from build123d import *

# Parameters (mm, degrees)
SKETCH1_W           = 121.3
SKETCH1_H           = 76.24
BOSS_EXTRUDE1_DEPTH = 7.4
SKETCH2_R           = 2.75
SKETCH2_R_2         = 1.5
BOSS_EXTRUDE2_DEPTH = 5.5
SKETCH3_R           = 2.75
SKETCH3_R_2         = 1.5
BOSS_EXTRUDE3_DEPTH = 5.3
SKETCH4_W           = 108
SKETCH4_H           = 65
CUT_EXTRUDE1_DEPTH  = 0.2
SKETCH5_R           = 8
BOSS_EXTRUDE4_DEPTH = 4
SKETCH6_W           = 5
SKETCH6_H           = 22
BOSS_EXTRUDE5_DEPTH = 3


with BuildPart() as part:
    # Sketch1 → Boss-Extrude1 (new body)
    with BuildSketch(Plane(origin=(0, 0, 0), x_dir=(1, 0, 0), z_dir=(0, 1, 0))):
        Rectangle(SKETCH1_W, SKETCH1_H)
    extrude(amount=BOSS_EXTRUDE1_DEPTH)

    # Sketch2 → Boss-Extrude2 (add)
    # profile 1 of 4: a face of its own
    with BuildSketch(Plane.XZ):
        with Locations(Location((-56.5, 34, 0), (0, 0, 270))):
            Circle(SKETCH2_R)
        with Locations(Location((-56.5, 34, 0), (0, 0, 270))):
            Circle(SKETCH2_R_2, mode=Mode.SUBTRACT)
    # profile 2 of 4: a face of its own
    with BuildSketch(Plane.XZ):
        with Locations(Location((56.5, 34, 0), (0, 0, 270))):
            Circle(SKETCH2_R)
        with Locations(Location((56.5, 34, 0), (0, 0, 270))):
            Circle(SKETCH2_R_2, mode=Mode.SUBTRACT)
    # profile 3 of 4: a face of its own
    with BuildSketch(Plane.XZ):
        with Locations(Location((56.5, -34, 0), (0, 0, 270))):
            Circle(SKETCH2_R)
        with Locations(Location((56.5, -34, 0), (0, 0, 270))):
            Circle(SKETCH2_R_2, mode=Mode.SUBTRACT)
    # profile 4 of 4: a face of its own
    with BuildSketch(Plane.XZ):
        with Locations(Location((-56.5, -34, 0), (0, 0, 270))):
            Circle(SKETCH2_R)
        with Locations(Location((-56.5, -34, 0), (0, 0, 270))):
            Circle(SKETCH2_R_2, mode=Mode.SUBTRACT)
    extrude(amount=BOSS_EXTRUDE2_DEPTH)

    # Sketch3 → Boss-Extrude3 (add)
    # profile 1 of 4: a face of its own
    with BuildSketch(Plane.XZ):
        with Locations(Location((-29.35, 24.62, 0), (0, 0, 270))):
            Circle(SKETCH3_R)
        with Locations(Location((-29.35, 24.62, 0), (0, 0, 270))):
            Circle(SKETCH3_R_2, mode=Mode.SUBTRACT)
    # profile 2 of 4: a face of its own
    with BuildSketch(Plane.XZ):
        with Locations(Location((28.65, 24.62, 0), (0, 0, 270))):
            Circle(SKETCH3_R)
        with Locations(Location((28.65, 24.62, 0), (0, 0, 270))):
            Circle(SKETCH3_R_2, mode=Mode.SUBTRACT)
    # profile 3 of 4: a face of its own
    with BuildSketch(Plane.XZ):
        with Locations(Location((28.65, -24.38, 0), (0, 0, 270))):
            Circle(SKETCH3_R)
        with Locations(Location((28.65, -24.38, 0), (0, 0, 270))):
            Circle(SKETCH3_R_2, mode=Mode.SUBTRACT)
    # profile 4 of 4: a face of its own
    with BuildSketch(Plane.XZ):
        with Locations(Location((-29.35, -24.38, 0), (0, 0, 270))):
            Circle(SKETCH3_R)
        with Locations(Location((-29.35, -24.38, 0), (0, 0, 270))):
            Circle(SKETCH3_R_2, mode=Mode.SUBTRACT)
    extrude(amount=BOSS_EXTRUDE3_DEPTH)

    # Sketch4 → Cut-Extrude1 (cut)
    with BuildSketch(Plane(origin=(0, 7.4, 0), x_dir=(1, 0, 0), z_dir=(0, 1, 0))):
        with Locations((0, 2.62)):
            Rectangle(SKETCH4_W, SKETCH4_H)
    extrude(amount=-CUT_EXTRUDE1_DEPTH, mode=Mode.SUBTRACT)

    # Sketch5 → Boss-Extrude4 (add)
    with BuildSketch(Plane(origin=(0, 0, 0), x_dir=(-1, 0, 0), z_dir=(0, -1, 0))):
        with Locations(Location((43.65, 30.12, 0), (0, 0, 90))):
            Circle(SKETCH5_R)
    extrude(amount=BOSS_EXTRUDE4_DEPTH)

    # Sketch6 → Boss-Extrude5 (add)
    with BuildSketch(Plane.XZ):
        with Locations((-45.15, -3.52)):
            Rectangle(SKETCH6_W, SKETCH6_H)
    extrude(amount=BOSS_EXTRUDE5_DEPTH)


solid = part.part
The model under review builds one solid part; all positions refer to its coordinate system, in mm. A direction names the side the tool comes from. Round coordinates to 2 decimals unless told otherwise and drop trailing zeros. Loops run counter-clockwise (first coordinate to the right, second up) from the corner with the lowest first, then second, coordinate; pieces in that order, holes last. Notation, with made-up numbers: (76, -4) - (117, -4) arc R15 ccw to (117, 24) - close; hole circle Ø3 at (29, 76). An arc over 180 degrees is marked (long way). Use CSV: the item, a comma, the result in double quotes.
(1) Take a section at D-D, the plane x = -29.35. Give the boundary of the cut face in (y, z).
Working result:
outline,"(-5.3, -27.13) - (0, -27.13) - (0, -38.12) - (7.4, -38.12) - (7.4, -35.12) - (7.2, -35.12) - (7.2, 29.88) - (7.4, 29.88) - (7.4, 38.12) - (0, 38.12) - (0, 27.37) - (-5.3, 27.37) - (-5.3, 26.12) - (0, 26.12) - (0, 23.12) - (-5.3, 23.12) - (-5.3, 21.87) - (0, 21.87) - (0, -21.63) - (-5.3, -21.63) - (-5.3, -22.88) - (0, -22.88) - (0, -25.88) - (-5.3, -25.88) - close"
(2) For line 1 (X direction, y = -2.7, z = 24.62); line 2 (X direction, y = -1.25, z = 35); line 3 (X direction, y = -1.55, z = -34), list the stretches that pass through material, from the lowest coordinate up.
Working result:
line 1,"x = -32.1 to -30.85, -27.85 to -26.6, 25.9 to 27.15, 30.15 to 31.4"
line 2,"x = -59.06 to -57.62, -55.38 to -53.94, 53.94 to 55.38, 57.62 to 59.06"
line 3,"x = -59.25 to -58, -55 to -53.75, -50.65 to -36.65, 53.75 to 55, 58 to 59.25"
(3) The part is to be moulded in two halves that separate along Z. For faces 1 (the flat face through (29, 0, -24)), 2 (the flat face through (-1, 4, 38.12)), 3 (the flat face through (60.65, 4, 1)), say which applies: pulls with the +Z half, pulls with the -Z half, needs draft (parallel to the pull), parting line crosses it, or undercut.
Working result:
face 1,"undercut"
face 2,"pulls with the +Z half"
face 3,"needs draft"
(4) Take a section at C-C, the plane z = 1. Give the boundary of the cut face in (x, y).
Working result:
outline,"(-60.65, 0) - (-47.65, 0) - (-47.65, -3) - (-42.65, -3) - (-42.65, 0) - (60.65, 0) - (60.65, 7.4) - (54, 7.4) - (54, 7.2) - (-54, 7.2) - (-54, 7.4) - (-60.65, 7.4) - close"
(5) Take a section at B-B, the plane x = -56.5. Give the boundary of the cut face in (y, z), plus the area to 3 significant figures.
Working result:
outline,"(-5.5, -36.75) - (0, -36.75) - (0, -38.12) - (7.4, -38.12) - (7.4, 38.12) - (0, 38.12) - (0, 36.75) - (-5.5, 36.75) - (-5.5, 35.5) - (0, 35.5) - (0, 32.5) - (-5.5, 32.5) - (-5.5, 31.25) - (0, 31.25) - (0, -31.25) - (-5.5, -31.25) - (-5.5, -32.5) - (0, -32.5) - (0, -35.5) - (-5.5, -35.5) - close"
area,"592 mm^2"
(6) Machinability: for faces 4 (the cylindrical face through (-29.925, -2.613, -25.766)), 5 (the flat face through (-9, 7.4, 31)), 6 (the flat face through (-47.65, -1, -4)), 7 (the flat face through (-1, 7.2, -3)), which of the approach directions +Z, -Z, +X, -X, +Y, -Y give a long, thin tool a straight path to every point of the face, cutting with its end or side? Answer none if there is none.
Working result:
face 4,"-Y"
face 5,"+Z, -Z, +X, -X, +Y"
face 6,"+Z, -X, -Y"
face 7,"+Y"
(7) Take a section at A-A, the plane y = -1.5. State how many separate pieces and enclosed holes the cut face has, plus the area to 3 significant figures.
Working result:
separate pieces,"10"
enclosed holes,"8"
area,"445 mm^2"
(8) Clearance check with flat-ended pins moving along their axes: P1, Ø1.5, axis at x = 29, z = 24.5, coming from the -Y side; P2, Ø0.9, axis at y = -1.5, z = -8, coming from the +X side; P3, Ø3, axis at x = -29, z = 25.5, coming from the -Y side. State where each tip first meets the part, or that it passes through.
Working result:
P1,"stops at y = 0"
P2,"stops at x = -42.65"
P3,"stops at y = -5.3"
